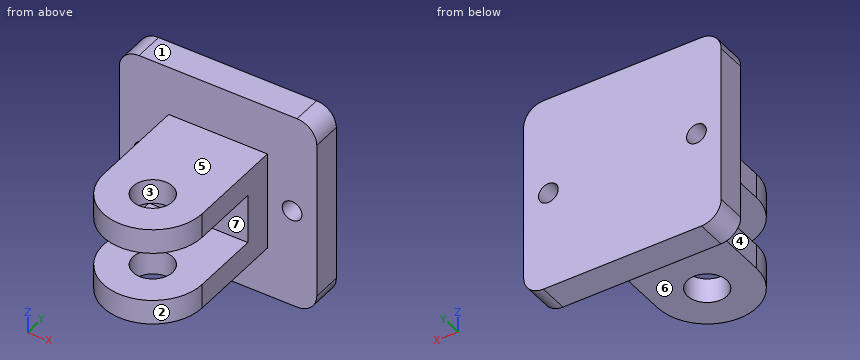
```python
from build123d import *

# Parameters (mm, degrees)
ESQUISSE1_W             = 10
ESQUISSE1_H             = 15
BOSS_EXTRU_1_DEPTH      = 10
CONG_1_RADIUS           = 5
CONG_1_LENGTH           = 10
ESQUISSE3_W             = 5
ESQUISSE3_H             = 12
ENL_V_MAT_EXTRU_1_DEPTH = 10
ESQUISSE4_W             = 10
ESQUISSE4_H             = 10
BOSS_EXTRU_2_DEPTH      = 3
ESQUISSE5_R             = 1
ENL_V_MAT_EXTRU_2_DEPTH = 3
ESQUISSE6_R             = 2
ENL_V_MAT_EXTRU_3_DEPTH = 21.862646045


with BuildPart() as part:
    # Esquisse1 → Boss.-Extru.1 (new body)
    with BuildSketch(Plane.XY):
        Rectangle(ESQUISSE1_W, ESQUISSE1_H)
    extrude(amount=BOSS_EXTRU_1_DEPTH)

    # Congé1: full round fillet: the end face becomes a half cylinder, R = half its width
    cong_1_face = Plane((0, -7.5, 5), x_dir=(0, 0, 1), z_dir=(0, -1, 0))  # on the end face: x along it, z out of the body
    cong_1_slab = cong_1_face.offset(-CONG_1_RADIUS / 2) * Box(CONG_1_LENGTH, 2 * CONG_1_RADIUS, CONG_1_RADIUS, mode=Mode.PRIVATE)  # the body's end, R deep
    cong_1_round = Plane((0, -2.5, 5), x_dir=(0, -1, 0), z_dir=(0, 0, 1)) * Cylinder(CONG_1_RADIUS, CONG_1_LENGTH, mode=Mode.PRIVATE)  # its axis R under the face
    add(cong_1_slab - cong_1_round, mode=Mode.SUBTRACT)

    # Esquisse3 → Enlèv. mat.-Extru.1 (cut)
    with BuildSketch(Plane.ZY.offset(5)):
        with Locations((5, -1.5)):
            Rectangle(ESQUISSE3_W, ESQUISSE3_H)
    extrude(amount=-ENL_V_MAT_EXTRU_1_DEPTH, mode=Mode.SUBTRACT)

    # Esquisse4 → Boss.-Extru.2 (add)
    # profile 1 of 2: a face of its own
    with BuildSketch(Plane(origin=(0, 7.5, 0), x_dir=(1, 0, 0), z_dir=(0, 1, 0))):
        with BuildLine():
            Line((8, 5), (-8, 5))
            ThreePointArc((-8, 5), (-9.414213562, 4.414213562), (-10, 3))
            Line((-10, 3), (-10, -13))
            ThreePointArc((-10, -13), (-9.414213562, -14.414213562), (-8, -15))
            Line((-8, -15), (8, -15))
            ThreePointArc((8, -15), (9.414213562, -14.414213562), (10, -13))
            Line((10, -13), (10, 3))
            ThreePointArc((10, 3), (9.414213562, 4.414213562), (8, 5))
        make_face()
        with Locations((0, -5)):
            Rectangle(ESQUISSE4_W, ESQUISSE4_H, mode=Mode.SUBTRACT)
    # profile 2 of 2: a face of its own
    with BuildSketch(Plane(origin=(0, 7.5, 0), x_dir=(1, 0, 0), z_dir=(0, 1, 0))):
        with Locations((0, -5)):
            Rectangle(ESQUISSE4_W, ESQUISSE4_H)
    extrude(amount=BOSS_EXTRU_2_DEPTH)

    # Esquisse5 → Enlèv. mat.-Extru.2 (cut)
    with BuildSketch(Plane.XZ.offset(-7.5)):
        with Locations(Location((-7.5, 5, 0), (0, 0, 270))):
            Circle(ESQUISSE5_R)
        with Locations(Location((7.5, 5, 0), (0, 0, 270))):
            Circle(ESQUISSE5_R)
    extrude(amount=-ENL_V_MAT_EXTRU_2_DEPTH, mode=Mode.SUBTRACT)

    # Esquisse6 → Enlèv. mat.-Extru.3 (cut, through all)
    with BuildSketch(Plane.XY.offset(10)):
        with Locations((0, -2.5)):
            Circle(ESQUISSE6_R)
    extrude(amount=-ENL_V_MAT_EXTRU_3_DEPTH, mode=Mode.SUBTRACT)


solid = part.part
```
Geometry check sheet. Reference: the model listing, model coordinates, mm. Face numbers are marked on the shaded views. A direction names the side the tool comes from. Coordinates: 2 decimals unless noted, no trailing zeros. Order: outer loops, then holes, each group sorted by start corner. A loop starts at its lowest first (then second) coordinate and runs counter-clockwise, first axis right, second up. Notation, with made-up numbers: M 58,-17.75 L 88,-17.75 A9 cw 88,-2.75 Z; hole C 9.25,-21.5 d4. An arc over 180 degrees is marked long. Answer as a JSON object with one key per item and string values.
Q1. Tool access check on the marked faces 4, 5, 6 and 7. Record the directions out of +Z, -Z, +X, -X, +Y, -Y that give a thin tool (end or side, any length) a straight path to the whole face; none if there is none.
Results are:
{"face 4": "+Z, -Z, -X, -Y", "face 5": "+Z, +X, -X, -Y", "face 6": "-Z, +X, -X, -Y", "face 7": "+X, -X, -Y"}
Q2. Cross-section at B-B on z = 5. Record the cut outline in (x, y).
Results are:
{"outline": "M -10,7.5 L -8.5,7.5 L -8.5,10.5 L -10,10.5 Z; M -6.5,7.5 L -5,7.5 L -5,4.5 L 5,4.5 L 5,7.5 L 6.5,7.5 L 6.5,10.5 L -6.5,10.5 Z; M 8.5,7.5 L 10,7.5 L 10,10.5 L 8.5,10.5 Z"}
Q3. Scan lines: line 1 (X direction, y = 8.5, z = 5); line 2 (Z direction, x = 4.75, y = 4.25); line 3 (Y direction, x = 0, z = 8.2). Record each from-to range of solid material in increasing order.
Results are:
{"line 1": "x = -10 to -8.5, -6.5 to 6.5, 8.5 to 10", "line 2": "z = 0 to 2.5, 7.5 to 10", "line 3": "y = -7.5 to -4.5, -0.5 to 10.5"}
Q4. Release check for a two-part mould opening along X. For the marked faces 1, 2 and 3 record: released by +X, released by -X, zero draft, split by the parting line, or undercut.
Results are:
{"face 1": "zero draft", "face 2": "split by the parting line", "face 3": "undercut"}
Q5. Cross-section at A-A on x = 0. Record the cut outline in (y, z).
Results are:
{"outline": "M -7.5,0 L -4.5,0 L -4.5,2.5 L -7.5,2.5 Z; M -7.5,7.5 L -4.5,7.5 L -4.5,10 L -7.5,10 Z; M -0.5,0 L 7.5,0 L 7.5,-5 L 10.5,-5 L 10.5,15 L 7.5,15 L 7.5,10 L -0.5,10 L -0.5,7.5 L 4.5,7.5 L 4.5,2.5 L -0.5,2.5 Z"}
Q6. Depth check by flat-ended pin: pin 1 Ø8 at (y, z) = (5, 0) entering from -X; pin 2 Ø3 at (x, y) = (0, 2) entering from +Z; pin 3 Ø1.2 at (x, z) = (-7.5, 5) entering from +Y; pin 4 Ø2 at (x, y) = (3, 0.5) entering from -Z. Enter the tip coordinate at first touch or a pass-through.
Results are:
{"pin 1": "stops at x = -10", "pin 2": "stops at z = 10", "pin 3": "passes through", "pin 4": "stops at z = 0"}
Q7. Cross-section at D-D on z = 1.75. Record the cut outline in (x, y), and give its area (3 significant figures).
Results are:
{"outline": "M -10,7.5 L -5,7.5 L -5,-2.5 A5 ccw 5,-2.5 L 5,7.5 L 10,7.5 L 10,10.5 L -10,10.5 Z; hole C 0,-2.5 d4", "area": "187 mm²"}
Q8. Cross-section at C-C on x = 7.5. Record the cut outline in (y, z), and give its area (3 significant figures).
Results are:
{"outline": "M 7.5,-5 L 10.5,-5 L 10.5,4 L 7.5,4 Z; M 7.5,6 L 10.5,6 L 10.5,15 L 7.5,15 Z", "area": "54.0 mm²"}
